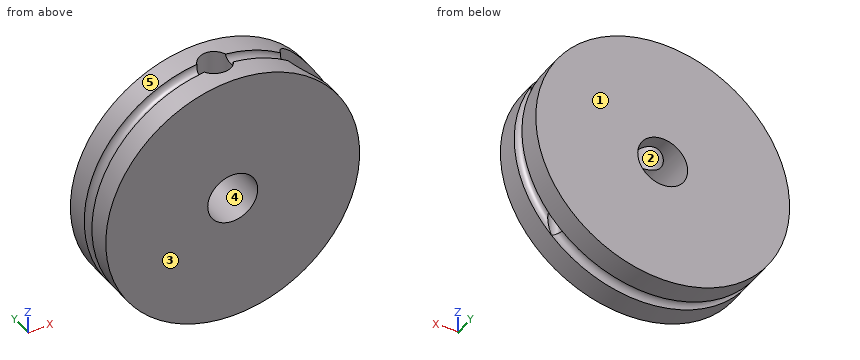
```python
from build123d import *

# Parameters (mm, degrees)
BASE_R                 = 12.7
BASE_R_2               = 2.5
MAIN_BODY_DEPTH        = 6
SKETCH4_R              = 0.65
CUT_EXTRUDE2_REACH     = 20.936
SKETCH5_R              = 1.58115
CUT_EXTRUDE3_START     = -8.980256222
CUT_EXTRUDE3_OUTLINE_R = 0.65
CUT_EXTRUDE3_DEPTH     = 17.960512444
SKETCH9_R              = 2.15
CUT_EXTRUDE4_DEPTH     = 19.936208868


# Read off the part's stored shape, not the designer's step: Cut-Extrude3
with BuildPart() as part:
    # BASE → MAIN_BODY (new body)
    with BuildSketch(Plane(origin=(0, 0, 0), x_dir=(1, 0, 0), z_dir=(0, 1, 0))):
        with Locations(Location((0, 0, 0), (0, 0, 270))):
            Circle(BASE_R)
        with Locations(Location((0, 0, 0), (0, 0, 270))):
            Circle(BASE_R_2, mode=Mode.SUBTRACT)
    extrude(amount=MAIN_BODY_DEPTH)

    # Sketch4 → CABLE_GUIDE (revolve, cut)
    with BuildSketch(Plane.XY):
        with Locations((12.7, 3)):
            Circle(SKETCH4_R)
    revolve(axis=Axis((0, 0, 0), (0, 1, 0)), mode=Mode.SUBTRACT)

    # Sketch5 → Cut-Extrude2 (cut, up to next)
    with BuildSketch(Plane.XY, mode=Mode.PRIVATE) as cut_extrude2_sk1:
        with Locations(Location((0, 3, 0), (0, 0, 180))):
            Circle(SKETCH5_R)
    cut_extrude2_tool1 = extrude(cut_extrude2_sk1.sketch, amount=CUT_EXTRUDE2_REACH, mode=Mode.PRIVATE) & part.part
    add(cut_extrude2_tool1.solids().sort_by_distance((0, 3, 0))[0], mode=Mode.SUBTRACT)

    # Cut-Extrude3 outline → Cut-Extrude3 (cut)
    with BuildSketch(Plane.XY.offset(CUT_EXTRUDE3_START)):
        with Locations((8.98025612, 3)):
            Circle(CUT_EXTRUDE3_OUTLINE_R)
    extrude(amount=CUT_EXTRUDE3_DEPTH, mode=Mode.SUBTRACT)

    # Sketch9 → Cut-Extrude4 (cut, through all)
    with BuildSketch(Plane.XY):
        with Locations(Location((8.98025612, 3, 0), (0, 0, 197.597336608))):
            Circle(SKETCH9_R)
    extrude(amount=CUT_EXTRUDE4_DEPTH, mode=Mode.SUBTRACT)


solid = part.part
```
Geometry check sheet. Reference: the model listing, model coordinates, mm. Face numbers are marked on the shaded views. A direction names the side the tool comes from. Give positions to 0.01 mm unless a question says otherwise; leave off trailing zeros. Write each loop counter-clockwise with the first axis right and the second up, starting at its lowest first coordinate (ties: lowest second). Pieces come first, ordered by that corner, then holes.
1) Material ranges on L1, parallel to X at y = 3.25, z = -1.75; L2, parallel to X at y = 3, z = 3.75; L3, parallel to X at y = 3, z = -6.5, recorded low to high.
2) Access from +Z, -Z, +X, -X, +Y, -Y to the whole of each face (thin tool, end or side, straight path). Record for the marked faces 1 and 2.
3) Section check A-A, the plane x = 0. Record the boundary of the cut face in (y, z), and give its area (3 significant figures).
4) Section check C-C, the plane z = -0.5. State how many separate pieces and enclosed holes the cut face has, and give its area (3 significant figures).
5) Section check D-D, the plane y = 5.5. Record the boundary of the cut face in (x, z), and give its area (3 significant figures).
6) Release check for a two-part mould opening along Z. For the marked faces 3, 4 and 5 record: pulls with the +Z half, pulls with the -Z half, needs draft (parallel to the pull), parting line crosses it, or undercut.
7) Section check B-B, the plane y = 3. Record the boundary of the cut face in (x, z), and give its area (3 significant figures).
8) Gauge pin test, flat ends, axial feed: pin 1 (6 mm diameter, centred on x = 9.5, z = 4.5, fed in from -Y); pin 2 (3.5 mm diameter, centred on x = 8.98, y = 3, fed in from -Z); pin 3 (1.5 mm diameter, centred on x = 1.5, y = 2, fed in from -Z); pin 4 (1 mm diameter, centred on x = 7, y = 4.5, fed in from -Z). Record the tip position at first contact, or that the pin passes through.
Computed:
1. L1: x = -11.97 to -1.79, 1.79 to 8.38, 9.58 to 11.97
1. L2: x = -11.45 to -1.58, 1.58 to 6.83, 11.13 to 11.45
1. L3: x = -10.15 to 8.33, 9.63 to 10.15
2. face 1: +Z, -Z, +X, -X, +Y
2. face 2: +Z
3. outline: (0, -12.7) - (2.35, -12.7) arc R0.65 cw to (3.65, -12.7) - (6, -12.7) - (6, -2.5) - (0, -2.5) - close; (0, 2.5) - (1.42, 2.5) - (1.42, 12.7) - (0, 12.7) - close; (4.58, 2.5) - (6, 2.5) - (6, 12.7) - (4.58, 12.7) - close
3. area: 89.5 mm2
4. separate pieces: 2
4. enclosed holes: 1
4. area: 120 mm2
5. outline: circle Ø25.4 at (0, 0); hole circle Ø5 at (0, 0)
5. area: 487 mm2
6. face 3: needs draft
6. face 4: undercut
6. face 5: parting line crosses it
7. outline: (-1.58, 1.94) - (-1.58, 11.95) arc R12.05 ccw (long way) to (8.33, -8.71) - (8.33, 0) - (6.83, 0) - (6.83, 9.93) arc R12.05 ccw to (1.58, 11.95) - (1.58, 1.94) arc R2.5 cw (long way) to start; (9.63, -7.24) arc R12.05 ccw to (11.13, 4.62) - (11.13, 0) - (9.63, 0) - close
7. area: 362 mm2
8. pin 1: stops at y = 0
8. pin 2: stops at z = -10.35
8. pin 3: stops at z = -12.68
8. pin 4: stops at z = -10.91
